Here's how the part is built. I have some questions about the finished solid (model axes, mm). Coordinates: 2 decimals unless noted, no trailing zeros. Loops run counter-clockwise (first coordinate to the right, second up) from the corner with the lowest first, then second, coordinate; pieces in that order, holes last.
```python
from build123d import *

# Parameters (mm, degrees)
F0_W     = 212.09
F0_H     = 25.4
F1_DEPTH = 12.7
F2_R     = 2.54
F4_W     = 7.62
F4_H     = 8.89
F5_DEPTH = 25.4


with BuildPart() as f1:
    # F0 (on Front) → F1 (new body)
    with BuildSketch(Plane.XZ):
        Rectangle(F0_W, F0_H)
    extrude(amount=F1_DEPTH)

    # F2
    f2_edges = [f1.edges().sort_by_distance(p)[0] for p in [
        (106.045, -6.35, 12.7),
        (106.045, -12.7, 0),
        (0, -12.7, 12.7),
        (0, -12.7, -12.7),
        (-106.045, -12.7, 0),
        (-106.045, -6.35, 12.7),
        (106.045, -6.35, -12.7),
        (-106.045, -6.35, -12.7),
    ]]
    fillet(f2_edges, radius=F2_R)

    # F4 (on Front) → F5 (cut)
    with BuildSketch(Plane.XZ):
        with Locations((94.615, 0)):
            Rectangle(F4_W, F4_H)
        with Locations((-94.615, 0)):
            Rectangle(F4_W, F4_H)
    extrude(amount=F5_DEPTH, mode=Mode.SUBTRACT)


solid = f1.part
```
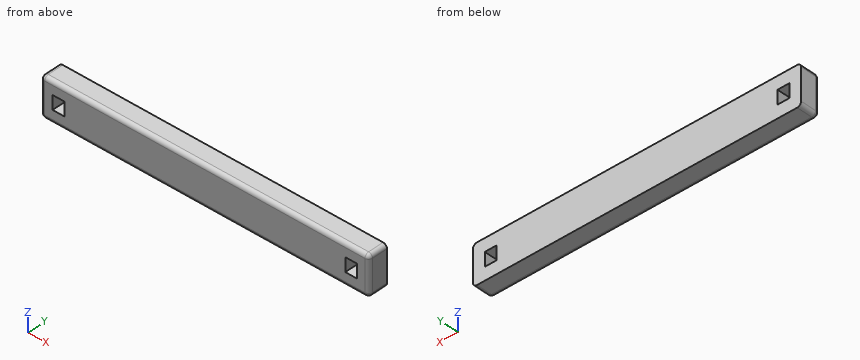
1. I need wall thicknesses on line 1 along X through (y, z) = (-5.25, -1) (3 decimals); line 2 along Z through (x, y) = (92.5, -1) (3 decimals); line 3 along X through (y, z) = (-11.75, 0.5) (3 decimals). Which ranges of each line are inside material? Lowest first, please.
2. I want a section at A-A (z = -1.25). Please give me the cut outline in (x, y) (3 decimals), then the cut area to 3 significant figures.
3. I want a section at B-B (y = -5.75). Please give me the cut outline in (x, z) (3 decimals), then the cut area to 3 significant figures.
Response values:
1. line 1: x = -106.045 to -98.425, -90.805 to 90.805, 98.425 to 106.045
1. line 2: z = -12.7 to -4.445, 4.445 to 12.7
1. line 3: x = -105.486 to -98.425, -90.805 to 90.805, 98.425 to 105.486
2. outline: (-106.045, -10.16) arc R2.54 ccw to (-103.505, -12.7) - (-98.425, -12.7) - (-98.425, 0) - (-106.045, 0) - close; (-90.805, -12.7) - (90.805, -12.7) - (90.805, 0) - (-90.805, 0) - close; (98.425, -12.7) - (103.505, -12.7) arc R2.54 ccw to (106.045, -10.16) - (106.045, 0) - (98.425, 0) - close
2. area: 2,500 mm2
3. outline: (-106.045, -10.16) arc R2.54 ccw to (-103.505, -12.7) - (103.505, -12.7) arc R2.54 ccw to (106.045, -10.16) - (106.045, 10.16) arc R2.54 ccw to (103.505, 12.7) - (-103.505, 12.7) arc R2.54 ccw to (-106.045, 10.16) - close; hole (-98.425, -4.445) - (-90.805, -4.445) - (-90.805, 4.445) - (-98.425, 4.445) - close; hole (90.805, -4.445) - (98.425, -4.445) - (98.425, 4.445) - (90.805, 4.445) - close
3. area: 5,250 mm2
